from build123d import *

# Parameters (mm, degrees)
BOSS_EXTRUDE1_DEPTH = 9
CUT_EXTRUDE1_DEPTH  = 25
BOSS_EXTRUDE2_DEPTH = 18
LPATTERN1_COUNT     = 5
LPATTERN1_PITCH     = 5
FILLET2_R           = 8
FILLET3_R           = 5
SKETCH6_R           = 1.5
CUT_EXTRUDE2_DEPTH  = 25
SKETCH7_W           = 12
SKETCH7_H           = 18.094661032
CUT_EXTRUDE3_DEPTH  = 8
SKETCH8_R           = 1.75
BOSS_EXTRUDE3_DEPTH = 1.5
SKETCH12_R          = 1.75
BOSS_EXTRUDE4_DEPTH = 1.5
CUT_EXTRUDE6_DEPTH  = 1.5


with BuildPart() as part:
    # Sketch3 → Boss-Extrude1 (new, symmetric)
    with BuildSketch(Plane(origin=(0, 0, 0), x_dir=(0, 0, -1), z_dir=(1, 0, 0))):
        with BuildLine():
            Line((49.79657451, 66.979899518), (70.136020437, 0))
            Line((70.136020437, 0), (65.359063047, -1.476711918))
            Line((65.359063047, -1.476711918), (66.429336182, -11.476711918))
            Line((66.429336182, -11.476711918), (75.217896234, -21.055919203))
            Line((75.217896234, -21.055919203), (84.07816774, -49.717663547))
            Line((84.07816774, -49.717663547), (84.07816774, -56.717663547))
            Line((84.07816774, -56.717663547), (95.07816774, -56.717663547))
            Line((95.07816774, -56.717663547), (95.07816774, -7.178658436))
            Line((95.07816774, -7.178658436), (102.149235552, -0.107590624))
            ThreePointArc((102.149235552, -0.107590624), (102.149235552, 8.37769075), (93.663954178, 8.37769075))
            Line((93.663954178, 8.37769075), (84.110365879, -1.175897549))
            Line((84.110365879, -1.175897549), (79.658453904, 3.276014426))
            Line((79.658453904, 3.276014426), (72.761111488, 73.953423835))
            Line((72.761111488, 73.953423835), (49.79657451, 66.979899518))
        make_face()
    extrude(amount=BOSS_EXTRUDE1_DEPTH, both=True)

    # Sketch4 → Cut-Extrude1 (cut)
    with BuildSketch(Plane(origin=(9, 0, 0), x_dir=(0, 0, -1), z_dir=(1, 0, 0))):
        Polygon((92.37816774, -49.772884049), (92.37816774, -24.772884049), (77.37816774, -24.772884049), align=None)
    extrude(amount=-CUT_EXTRUDE1_DEPTH, mode=Mode.SUBTRACT)

    # Sketch5 → Boss-Extrude2 (add)
    with BuildSketch(Plane(origin=(9, 0, 0), x_dir=(0, 0, -1), z_dir=(1, 0, 0))):
        Polygon((95.07816774, -47.717663547), (95.07816774, -49.717663547), (99.07816774, -49.717663547), align=None)
        Polygon((99.07816774, -49.717663547), (95.07816774, -49.717663547), (95.07816774, -51.717663547), align=None)
    boss_extrude2 = extrude(amount=-BOSS_EXTRUDE2_DEPTH)

    # LPattern1: Boss-Extrude2 ×5
    with Locations(*[(0, i * LPATTERN1_PITCH, 0) for i in range(1, LPATTERN1_COUNT)]):
        add(boss_extrude2)

    # Fillet2
    # the kernel refuses this fillet: 8 mm, written as the material it takes off along each edge
    with BuildSketch(Plane(origin=(-15.580741663, -11.476711918, -66.429336182), x_dir=(0, 0.9943213171006763, 0.10641953936743088), z_dir=(1, 0, 0))) as fillet2_piece_1:
        with BuildLine():
            CenterArc((FILLET2_R * 0.329037083141, -FILLET2_R), FILLET2_R, 90, 36.426245441)
            Line((-FILLET2_R * 0.264750438373, -FILLET2_R * 0.195378114085), (-FILLET2_R * 0.276626188803, -FILLET2_R * 0.179285676366))
            Line((-FILLET2_R * 0.276626188803, -FILLET2_R * 0.179285676366), (-FILLET2_R * 0.00658074166282, FILLET2_R * 0.02))
            Line((-FILLET2_R * 0.00658074166282, FILLET2_R * 0.02), (FILLET2_R * 0.329037083141, FILLET2_R * 0.02))
            Line((FILLET2_R * 0.329037083141, FILLET2_R * 0.02), (FILLET2_R * 0.329037083141, 0))
        make_face()
    extrude(amount=31.161483326, mode=Mode.SUBTRACT)
    with BuildSketch(Plane(origin=(-25.044809619, -1.476711918, -65.359063047), x_dir=(0, 0.2953423835382918, -0.9553914781313054), z_dir=(1, 0, 0))) as fillet2_piece_2:
        with BuildLine():
            CenterArc((6.618974651, -7.834470057), FILLET2_R, 101.675691656, 67.255197487)
            Line((-1.232195855, -6.298526803), (-1.389219265, -6.267807938))
            Line((-1.389219265, -6.267807938), (-0.15702341, 0.030718865))
            Line((-0.15702341, 0.030718865), (0, 0.16))
            ThreePointArc((0, 0.16), (2.5, 0.16), (4.967620507, 0.156689401))
            Line((4.967620507, 0.156689401), (5, 0))
        make_face()
    extrude(amount=50.089619238, mode=Mode.SUBTRACT)

    # Fillet3
    fillet3_edges = [part.edges().sort_by_distance(p)[0] for p in [
        (0, 66.979899518, -49.79657451),
        (0, 73.953423835, -72.761111488),
    ]]
    fillet(fillet3_edges, radius=FILLET3_R)

    # Sketch6 → Cut-Extrude2 (cut)
    with BuildSketch(Plane(origin=(9, 0, 0), x_dir=(0, 0, -1), z_dir=(1, 0, 0))):
        with Locations((56.033670614, 63.648438547)):
            Circle(SKETCH6_R)
    extrude(amount=-CUT_EXTRUDE2_DEPTH, mode=Mode.SUBTRACT)

    # Sketch7 → Cut-Extrude3 (cut)
    with BuildSketch(Plane(origin=(0, 19.387405719, -62.715557398), x_dir=(1, 0, 0), z_dir=(0, -0.29534238353829306, 0.955391478131305))):
        with Locations((0, -58.879009045)):
            Rectangle(SKETCH7_W, SKETCH7_H)
    extrude(amount=-CUT_EXTRUDE3_DEPTH, mode=Mode.SUBTRACT)

    # Sketch8 → Boss-Extrude3 (add)
    with BuildSketch(Plane(origin=(9, 0, 0), x_dir=(0, 0, -1), z_dir=(1, 0, 0))):
        with Locations((97.906594865, 4.135050063)):
            Circle(SKETCH8_R)
    boss_extrude3 = extrude(amount=BOSS_EXTRUDE3_DEPTH)

    # Sketch12 → Boss-Extrude4 (add)
    with BuildSketch(Plane(origin=(9, 0, 0), x_dir=(0, 0, -1), z_dir=(1, 0, 0))):
        with Locations((73.996626083, -7.006834096)):
            Circle(SKETCH12_R)
    boss_extrude4 = extrude(amount=BOSS_EXTRUDE4_DEPTH)

    # Sketch13 → Cut-Extrude6 (cut)
    with BuildSketch(Plane(origin=(9, 0, 0), x_dir=(0, 0, -1), z_dir=(1, 0, 0))):
        with BuildLine():
            Line((73.173071484, 13.27485534), (73.467077668, 13.955552183))
            ThreePointArc((73.467077668, 13.955552183), (73.53702701, 14.197471144), (73.544321074, 14.449194188))
            Line((73.544321074, 14.449194188), (68.990982491, 61.107480203))
            ThreePointArc((68.990982491, 61.107480203), (68.551531185, 61.841654795), (67.705147046, 61.967208252))
            Line((67.705147046, 61.967208252), (58.443343887, 59.154723523))
            ThreePointArc((58.443343887, 59.154723523), (57.851848811, 58.669007544), (57.777051693, 57.907304302))
            Line((57.777051693, 57.907304302), (71.298187251, 13.380806172))
            ThreePointArc((71.298187251, 13.380806172), (72.198622375, 12.672962595), (73.173071484, 13.27485534))
        make_face()
    cut_extrude6 = extrude(amount=-CUT_EXTRUDE6_DEPTH, mode=Mode.SUBTRACT)

    # Mirror1: Boss-Extrude3, Boss-Extrude4, Cut-Extrude6 across plane
    add(boss_extrude3.mirror(Plane(origin=(0, 0, 0), x_dir=(0, 0, 1), z_dir=(1, 0, 0))))
    add(boss_extrude4.mirror(Plane(origin=(0, 0, 0), x_dir=(0, 0, 1), z_dir=(1, 0, 0))))
    add(cut_extrude6.mirror(Plane(origin=(0, 0, 0), x_dir=(0, 0, 1), z_dir=(1, 0, 0))), mode=Mode.SUBTRACT)


solid = part.part
Geometry: final body of the model. Coordinates: model frame, mm. A direction names the side the tool comes from. Give positions to 0.01 mm unless a question says otherwise; leave off trailing zeros. Write each loop counter-clockwise with the first axis right and the second up, starting at its lowest first coordinate (ties: lowest second). Pieces come first, ordered by that corner, then holes.
(1) Mould query, pull axis Z, two halves, no side actions, for faces 5 (the flat face through (-10.5, -7, -74)), 6 (the cylindrical face through (0.126, 8.283, -102.242)), 7 (the flat face through (-8.26, 35.96, -64.44)), 8 (the flat face through (0.13, -45.73, -97.05)). Classes: released by +Z, released by -Z, zero draft, split by the parting line, or undercut.
(2) Cut plane B-B, the plane z = -63. Return loops of the section in (x, y), then the cut area to 3 significant figures.
(3) Ray query, line 1 (X direction, y = -42, z = -83); line 2 (Y direction, x = 3.25, z = -88.5); line 3 (X direction, y = -39.5, z = -94.5). Return the intervals inside material, ascending.
(4) Access query for faces 1 (the flat face through (-8.26, 60.58, -63.14)), 2 (the flat face through (7.5, 43, -67)), 3 (the flat face through (0.126, 1.019, -81.916)), 4 (the flat face through (0.126, -38.732, -97.106)). Directions: +Z, -Z, +X, -X, +Y, -Y. A direction counts if a zero-diameter tool reaches every point of the face in a straight line with its end or side. Return the directions, or none.
(5) Cut plane C-C, the plane y = -10. Return loops of the section in (x, z).
(6) Cut plane A-A, the plane y = 34.5. Return loops of the section in (x, z), then the cut area to 3 significant figures.
(7) First-contact query: P1, Ø2, axis at x = 0.5, z = -90.5, coming from the +Y side; P2, Ø8, axis at y = 47, z = -66, coming from the -X side; P3, Ø5.5, axis at x = 4, y = -15, coming from the -Z side; P4, Ø2.5, axis at y = 63.65, z = -56.03, coming from the +X side. Flat tips, straight axial feed; report the tip coordinate or a pass-through.
Values follow:
1. face 5: zero draft
1. face 6: undercut
1. face 7: undercut
1. face 8: released by -Z
2. outline: (-9, 23.5) - (9, 23.5) - (9, 40.71) - (7.5, 40.71) - (7.5, 60.54) - (9, 60.54) - (9, 70.99) - (-9, 70.99) - (-9, 60.54) - (-7.5, 60.54) - (-7.5, 40.71) - (-9, 40.71) - close
2. area: 795 mm2
3. line 1: x = -9 to -6, 6 to 9
3. line 2: y = -56.72 to -43.74, -24.77 to 3.21
3. line 3: x = -9 to 9
4. face 1: -X
4. face 2: +X
4. face 3: +X, -X, +Y
4. face 4: -Z, +X, -X
5. outline: (-9, -95.08) - (9, -95.08) - (9, -66.36) - (-9, -66.36) - close
6. outline: (-9, -76.61) - (9, -76.61) - (9, -71.59) - (7.5, -71.59) - (7.5, -64.89) - (9, -64.89) - (9, -59.66) - (-9, -59.66) - (-9, -64.89) - (-7.5, -64.89) - (-7.5, -71.59) - (-9, -71.59) - close
6. area: 285 mm2
7. P1: stops at y = 6.21
7. P2: stops at x = -7.5
7. P3: stops at z = -95.08
7. P4: passes through
